Answer from the drawing. Dimensions are ordinates in mm from the lowest x, y and z of the part. Give positions to 0.01 mm unless a question says otherwise; leave off trailing zeros. Write each loop counter-clockwise with the first axis right and the second up, starting at its lowest first coordinate (ties: lowest second). Pieces come first, ordered by that corner, then holes. Notation, with made-up numbers: (-29.5, 52.25) -> (20.5, 52.25) arc R23 cw to (20.5, 68.25) -> close; hole circle Ø4 at (-28.75, -15.75). An arc over 180 degrees is marked (long way). Use a Markdown table: item, result. Add a question column.
Q1. Section A-A, the plane y = 4.1 is taken. Give the vertices of the cut face in (x, z).
Q2. Consider line 1 (X direction, y = 1.1, z = 10); line 2 (Z direction, x = 140, y = 1.35); line 3 (X direction, y = 3, z = 7). Determine where each line is inside the solid, lowest interval first.
Q3. This flat-tipped pin is pushed along its axis until it touches: pin 1 Ø3.5 at (x, z) = (140, 30) entering from -Y. Where does it stop, or does it pass through?
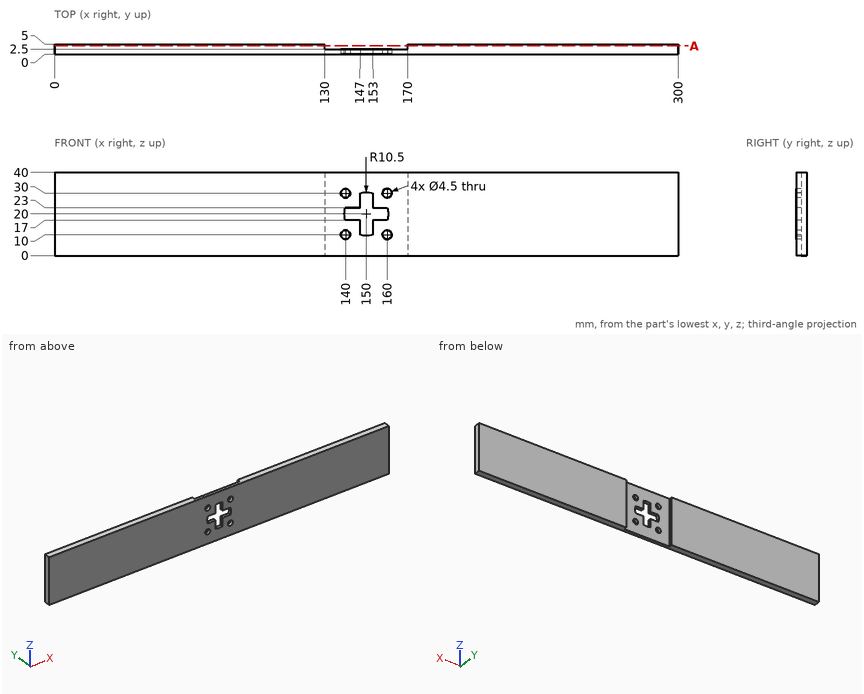
Result set:
| question | item | result |
|---|---|---|
| 1 | outline | (0, 0) -> (130, 0) -> (130, 40) -> (0, 40) -> close; (170, 0) -> (300, 0) -> (300, 40) -> (170, 40) -> close |
| 2 | line 1 | x = 0 to 137.75, 142.25 to 147, 153 to 157.75, 162.25 to 300 |
| 2 | line 2 | z = 0 to 7.75, 12.25 to 17, 23 to 27.75, 32.25 to 40 |
| 2 | line 3 | x = 0 to 130, 170 to 300 |
| 3 | pin 1 | passes through |
